Work out the finished part from the listing and answer in its coordinate system (mm). A direction names the side the tool comes from. Round coordinates to 2 decimals unless told otherwise and drop trailing zeros. Order: outer loops, then holes, each group sorted by start corner. A loop starts at its lowest first (then second) coordinate and runs counter-clockwise, first axis right, second up. Notation, with made-up numbers: (46, 43) -> (70, 43) arc R30 cw to (70, 66) -> close; hole circle Ø11 at (81.25, -15). An arc over 180 degrees is marked (long way). Use a Markdown table: item, result. Add a question column.
Item 1: For a pull along Z with two mould halves and no side action, classify faces 6 (the cylindrical face through (-11.93, 35.5, -0.48)), 7 (the flat face through (-12.2, 34.925, 0.1)), 8 (the flat face through (10, 14, -3.175)) as +Z half, -Z half, draft (parallel to the pull), parting line (faces both ways), or undercut.
Item 2: A cutting plane is placed at B-B, the plane z = 0. Determine the outline of the cut face in (x, y) (3 decimals), plus the area to 3 significant figures.
Item 3: A cutting plane is placed at D-D, the plane x = -9.5. Determine the outline of the cut face in (y, z) (3 decimals), plus the area to 3 significant figures.
Item 4: Find the intervals of material crossed by L1, parallel to Z at x = 0, y = 3 (3 decimals); L2, parallel to Z at x = 0, y = 21.5; L3, parallel to Y at x = -14, z = 10.5, in increasing order. Write a range as [from, to].
Item 5: A cutting plane is placed at A-A, the plane x = 0. Determine the outline of the cut face in (y, z) (3 decimals).
Item 6: A tool of negligible diameter and unlimited length cuts with its end or side. For faces 1 (the cylindrical face through (-27.28, 2.5, -1.16)), 2 (the flat face through (0, 0, 6)), 3 (the flat face through (12, 5.08, 12)), 4 (the flat face through (-12.2, 36.093, 0.1)), 5 (the flat face through (10, 14, 3.175)), from which of +Z, -Z, +X, -X, +Y, -Y can it reach the whole face along a straight path? Write none if from no direction.
Item 7: Flat-ended cylindrical pins translate along their axes: P1, Ø1, axis at x = -17.5, z = 8, coming from the +Y side; P2, Ø7, axis at x = 10.5, y = 25.5, coming from the +Z side; P3, Ø12, axis at y = 23.5, z = -6, coming from the -X side. Find the tip coordinate at first contact, or state that the pin passes through.
Item 8: A cutting plane is placed at C-C, the plane y = 27. Determine the outline of the cut face in (x, z) (3 decimals).
from build123d import *

# Parameters (mm, degrees)
SKETCH1_R           = 27.305
SKETCH1_R_2         = 4.5466
BOSS_EXTRUDE1_DEPTH = 50.8
SKETCH2_R           = 6.35
CUT_EXTRUDE1_DEPTH  = 44.45
SKETCH3_OUTSIDE_W   = 75.098
SKETCH3_OUTSIDE_H   = 75.098
SKETCH3_OUTSIDE_R   = 12.7
CUT_EXTRUDE2_DEPTH  = 44.45
SKETCH10_W          = 30.679481275
SKETCH10_H          = 6.35
CUT_EXTRUDE7_DEPTH  = 6.35
SKETCH13_OUTSIDE_W  = 74.891
SKETCH13_OUTSIDE_H  = 75.076
SKETCH13_OUTSIDE_R  = 11.938
CUT_EXTRUDE9_DEPTH  = 1.1684
SKETCH16_R          = 46.08237905
CUT_EXTRUDE11_DEPTH = 14.335
SKETCH18_R          = 16.51
SKETCH18_R_2        = 12.7
BOSS_EXTRUDE4_DEPTH = 3.81
SKETCH19_OUTSIDE_W  = 73.569
SKETCH19_OUTSIDE_H  = 73.754
SKETCH19_OUTSIDE_R  = 16.51
CUT_EXTRUDE12_DEPTH = 1.27
SKETCH10_2_W        = 30.679481275
SKETCH10_2_H        = 6.35
CUT_EXTRUDE13_DEPTH = 38.465


with BuildPart() as part:
    # Sketch1 → Boss-Extrude1 (new body)
    with BuildSketch(Plane(origin=(0, 0, 0), x_dir=(1, 0, 0), z_dir=(0, 1, 0))):
        Circle(SKETCH1_R)
        Circle(SKETCH1_R_2, mode=Mode.SUBTRACT)
    extrude(amount=BOSS_EXTRUDE1_DEPTH)

    # Sketch2 → Cut-Extrude1 (cut)
    with BuildSketch(Plane(origin=(0, 50.8, 0), x_dir=(1, 0, 0), z_dir=(0, 1, 0))):
        Circle(SKETCH2_R)
    extrude(amount=-CUT_EXTRUDE1_DEPTH, mode=Mode.SUBTRACT)

    # Sketch3 outside → Cut-Extrude2 (cut)
    with BuildSketch(Plane(origin=(0, 50.8, 0), x_dir=(1, 0, 0), z_dir=(0, 1, 0))):
        Rectangle(SKETCH3_OUTSIDE_W, SKETCH3_OUTSIDE_H)
        Circle(SKETCH3_OUTSIDE_R, mode=Mode.SUBTRACT)
    extrude(amount=-CUT_EXTRUDE2_DEPTH, mode=Mode.SUBTRACT)

    # Sketch10 → Cut-Extrude7 (cut)
    with BuildSketch(Plane.XZ):
        with Locations((17.839550223, 0)):
            Rectangle(SKETCH10_W, SKETCH10_H)
    extrude(amount=-CUT_EXTRUDE7_DEPTH, mode=Mode.SUBTRACT)

    # Sketch13 outside → Cut-Extrude9 (cut)
    with BuildSketch(Plane(origin=(0, 34.925, 0), x_dir=(-1, 0, 0), z_dir=(0, 1, 0))):
        with Locations((0.0925, 0)):
            Rectangle(SKETCH13_OUTSIDE_W, SKETCH13_OUTSIDE_H)
        Circle(SKETCH13_OUTSIDE_R, mode=Mode.SUBTRACT)
    extrude(amount=CUT_EXTRUDE9_DEPTH, mode=Mode.SUBTRACT)

    # Sketch16 → Cut-Extrude11 (cut, through all)
    with BuildSketch(Plane(origin=(0, 37.465, 0), x_dir=(-1, 0, 0), z_dir=(0, 1, 0))):
        Circle(SKETCH16_R)
    extrude(amount=CUT_EXTRUDE11_DEPTH, mode=Mode.SUBTRACT)

    # Sketch18 → Boss-Extrude4 (add)
    with BuildSketch(Plane(origin=(0, 6.35, 0), x_dir=(1, 0, 0), z_dir=(0, 1, 0))):
        Circle(SKETCH18_R)
        Circle(SKETCH18_R_2, mode=Mode.SUBTRACT)
    extrude(amount=BOSS_EXTRUDE4_DEPTH)

    # Sketch19 outside → Cut-Extrude12 (cut)
    with BuildSketch(Plane(origin=(0, 6.35, 0), x_dir=(1, 0, 0), z_dir=(0, 1, 0))):
        with Locations((-0.0925, 0)):
            Rectangle(SKETCH19_OUTSIDE_W, SKETCH19_OUTSIDE_H)
        Circle(SKETCH19_OUTSIDE_R, mode=Mode.SUBTRACT)
    extrude(amount=-CUT_EXTRUDE12_DEPTH, mode=Mode.SUBTRACT)

    # Sketch10_2 → Cut-Extrude13 (cut, through all)
    with BuildSketch(Plane.XZ):
        with Locations((17.839550223, 0)):
            Rectangle(SKETCH10_2_W, SKETCH10_2_H)
    extrude(amount=-CUT_EXTRUDE13_DEPTH, mode=Mode.SUBTRACT)


solid = part.part
Reported:
| question | item | result |
|---|---|---|
| 1 | face 6 | parting line |
| 1 | face 7 | draft |
| 1 | face 8 | undercut |
| 2 | outline | (-27.305, 0) -> (-4.547, 0) -> (-4.547, 6.35) -> (-6.35, 6.35) -> (-6.35, 37.465) -> (-12.7, 37.465) -> (-12.7, 36.093) -> (-11.938, 36.093) -> (-11.938, 34.925) -> (-12.7, 34.925) -> (-12.7, 10.16) -> (-16.51, 10.16) -> (-16.51, 5.08) -> (-27.305, 5.08) -> close |
| 2 | area | 342 mm² |
| 3 | outline | (0, -25.599) -> (5.08, -25.599) -> (5.08, -13.503) -> (10.16, -13.503) -> (10.16, -8.429) -> (34.925, -8.429) -> (34.925, -7.23) -> (36.093, -7.23) -> (36.093, -8.429) -> (37.465, -8.429) -> (37.465, 8.429) -> (36.093, 8.429) -> (36.093, 7.23) -> (34.925, 7.23) -> (34.925, 8.429) -> (10.16, 8.429) -> (10.16, 13.503) -> (5.08, 13.503) -> (5.08, 25.599) -> (0, 25.599) -> close |
| 3 | area | 855 mm² |
| 4 | L1 | [-27.305, -4.547], [4.547, 27.305] |
| 4 | L2 | [-12.7, -6.35], [6.35, 12.7] |
| 4 | L3 | [0, 5.08] |
| 5 | outline | (0, -27.305) -> (5.08, -27.305) -> (5.08, -16.51) -> (10.16, -16.51) -> (10.16, -12.7) -> (34.925, -12.7) -> (34.925, -11.938) -> (36.093, -11.938) -> (36.093, -12.7) -> (37.465, -12.7) -> (37.465, -6.35) -> (6.35, -6.35) -> (6.35, -4.547) -> (0, -4.547) -> close; (0, 4.547) -> (6.35, 4.547) -> (6.35, 6.35) -> (37.465, 6.35) -> (37.465, 12.7) -> (36.093, 12.7) -> (36.093, 11.938) -> (34.925, 11.938) -> (34.925, 12.7) -> (10.16, 12.7) -> (10.16, 16.51) -> (5.08, 16.51) -> (5.08, 27.305) -> (0, 27.305) -> close |
| 6 | face 1 | +Y, -Y |
| 6 | face 2 | +Z, -Z, +X, -X, -Y |
| 6 | face 3 | +Y |
| 6 | face 4 | none |
| 6 | face 5 | +X, +Y, -Y |
| 7 | P1 | y = 5.08 |
| 7 | P2 | z = 10.6 |
| 7 | P3 | x = -12.7 |
| 8 | outline | (5.499, -3.175) arc R6.35 cw (long way) to (5.499, 3.175) -> (12.297, 3.175) arc R12.7 ccw (long way) to (12.297, -3.175) -> close |
